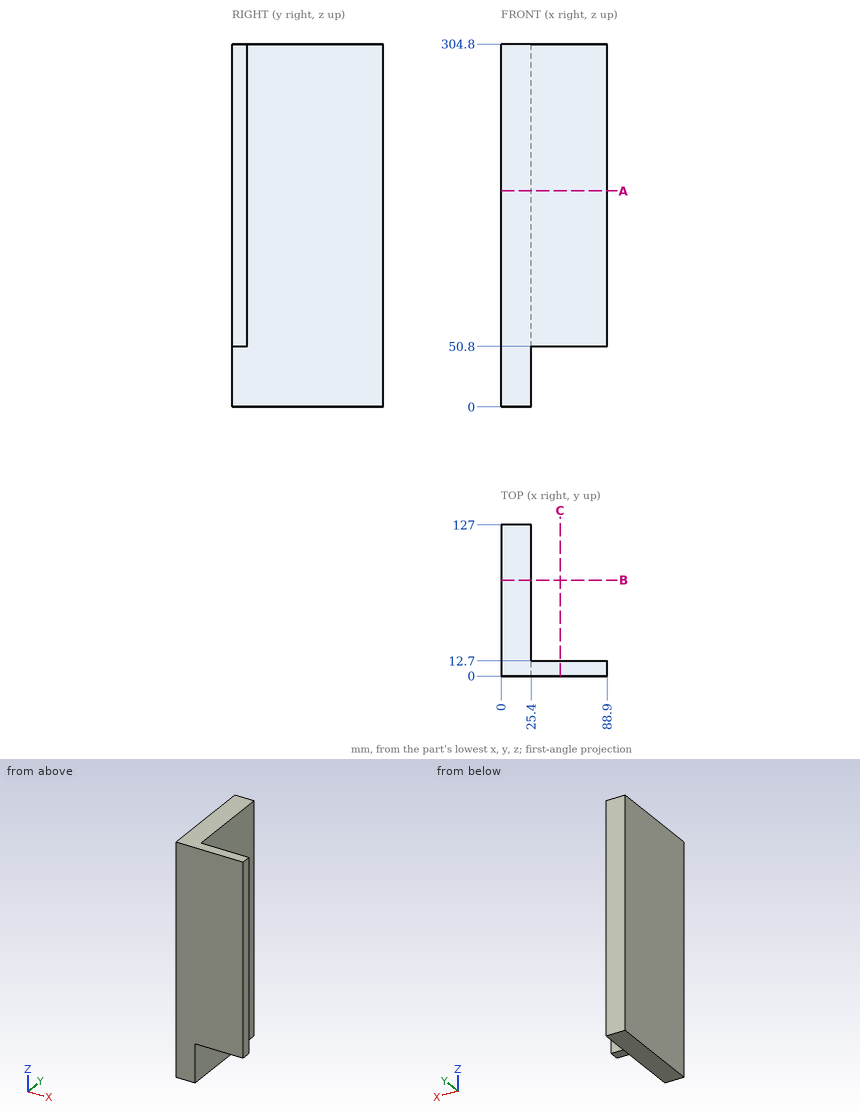
Verification items for this drawing (mm, ordinates from the low corner). Coordinates: 2 decimals unless noted, no trailing zeros. Order: outer loops, then holes, each group sorted by start corner. A loop starts at its lowest first (then second) coordinate and runs counter-clockwise, first axis right, second up. Notation, with made-up numbers: (-13, -17.5) - (3, -17.5) arc R12 cw to (3, 3.5) - close; hole circle Ø7 at (51, 20.5). An arc over 180 degrees is marked (long way). Answer as a JSON object with one key per item and string values. Group by question number.
Item 1: Scan lines: probe 1 along X at (y, z) = (57, 236); probe 2 along Y at (x, z) = (57, 229). Record each from-to range of solid material in increasing order.
Item 2: Sectioned sample at B-B, the plane y = 80.5. Record the cut outline in (x, z), and give its area (3 significant figures).
Item 3: Sectioned sample at C-C, the plane x = 49.5. Record the cut outline in (y, z), and give its area (3 significant figures).
Item 4: Sectioned sample at A-A, the plane z = 181.5. Record the cut outline in (x, y), and give its area (3 significant figures).
Item 5: Depth check by flat-ended pin: pin 1 Ø10 at (y, z) = (86.5, 57) entering from +X; pin 2 Ø3 at (y, z) = (41.5, 90.5) entering from -X; pin 3 Ø6.5 at (x, y) = (58.5, 4) entering from -Z. Enter the tip coordinate at first touch or a pass-through.
Resolved:
{
 "1": {"probe 1": "0 to 25.4", "probe 2": "0 to 12.7"},
 "2": {"outline": "(0, 0) - (25.4, 0) - (25.4, 304.8) - (0, 304.8) - close", "area": "7,740 mm^2"},
 "3": {"outline": "(0, 50.8) - (12.7, 50.8) - (12.7, 304.8) - (0, 304.8) - close", "area": "3,230 mm^2"},
 "4": {"outline": "(0, 0) - (88.9, 0) - (88.9, 12.7) - (25.4, 12.7) - (25.4, 127) - (0, 127) - close", "area": "4,030 mm^2"},
 "5": {"pin 1": "x = 25.4", "pin 2": "x = 0", "pin 3": "z = 50.8"}
}
